Can you work these out from the model? Positions are in its coordinate system, mm. A direction names the side the tool comes from. Round coordinates to 2 decimals unless told otherwise and drop trailing zeros. Order: outer loops, then holes, each group sorted by start corner. A loop starts at its lowest first (then second) coordinate and runs counter-clockwise, first axis right, second up. Notation, with made-up numbers: (24, 53) -> (74, 53) arc R22 cw to (74, 68) -> close; hole circle Ø8 at (43.25, 3). An arc over 180 degrees is marked (long way). One line per item, written item: value.
```python
from build123d import *

# Parameters (mm, degrees)
F1_DEPTH    = 3
F3_DEPTH    = 6
F5_DEPTH    = 12.5
F6_W        = 30
F6_H        = 2.0356480181
F7_DEPTH    = 8
F8_T4_DEPTH = 30
F8_T9_DEPTH = 30


# Not quite as in the source:
# - a fillet or chamfer that OpenCascade refuses, or shapes differently, is made with other operations: its cross-section is extruded or revolved along the edge and cut away or added


with BuildPart() as f1:
    # F0 (on Top) → F1 (new body)
    with BuildSketch(Plane.XY):
        with BuildLine():
            ThreePointArc((22, 30), (20.5355339059, 33.5355339059), (17, 35))
            Line((17, 35), (-17, 35))
            ThreePointArc((-17, 35), (-20.5355339059, 33.5355339059), (-22, 30))
            Line((-22, 30), (-22, -30))
            ThreePointArc((-22, -30), (-20.5355339059, -33.5355339059), (-17, -35))
            Line((-17, -35), (17, -35))
            ThreePointArc((17, -35), (20.5355339059, -33.5355339059), (22, -30))
            Line((22, -30), (22, 30))
        make_face()
    extrude(amount=F1_DEPTH)

    # F2 (on Top) → F3 (join)
    with BuildSketch(Plane.XY):
        with BuildLine():
            ThreePointArc((-12, 30), (-13.4644661049, 33.5355339167), (-17.0000000305, 35))
            ThreePointArc((-17.0000000305, 35), (-20.5355339275, 33.5355338843), (-22, 29.9999999695))
            ThreePointArc((-22, 29.9999999695), (-16.9999999847, 25), (-12, 30))
        make_face()
        with BuildLine():
            ThreePointArc((22, 30), (20.5355339059, 33.5355339059), (17, 35))
            ThreePointArc((17, 35), (13.4644660941, 26.4644660941), (22, 30))
        make_face()
        with BuildLine():
            ThreePointArc((17, -35), (20.5355339059, -33.5355339059), (22, -30))
            ThreePointArc((22, -30), (13.4644660941, -26.4644660941), (17, -35))
        make_face()
        with BuildLine():
            ThreePointArc((-12, -30), (-17, -25), (-22, -30))
            ThreePointArc((-22, -30), (-20.5355339059, -33.5355339059), (-17, -35))
            ThreePointArc((-17, -35), (-13.4644660941, -33.5355339059), (-12, -30))
        make_face()
    extrude(amount=F3_DEPTH)

    # F4 (on Top) → F5 (cut, symmetric)
    with BuildSketch(Plane.XY):
        with BuildLine():
            ThreePointArc((-18.0685374254, -32.3153245497), (-15.6256402281, -32.1479374333), (-14.45, -30))
            ThreePointArc((-14.45, -30), (-14.5093597608, -29.4529979899), (-14.6846754503, -28.9314625746))
            Line((-14.6846754503, -28.9314625746), (-18.0685374254, -32.3153245497))
        make_face()
        with BuildLine():
            Line((-18.0685374254, -32.3153245497), (-14.6846754503, -28.9314625746))
            ThreePointArc((-14.6846754503, -28.9314625746), (-15.196877708, -28.196877708), (-15.9314625746, -27.6846754503))
            Line((-15.9314625746, -27.6846754503), (-19.3153245497, -31.0685374254))
            ThreePointArc((-19.3153245497, -31.0685374254), (-18.803122292, -31.803122292), (-18.0685374254, -32.3153245497))
        make_face()
        with BuildLine():
            ThreePointArc((-15.9314625746, -27.6846754503), (-15.196877708, -28.196877708), (-14.6846754503, -28.9314625746))
            Line((-14.6846754503, -28.9314625746), (-14.16467731, -28.4114644343))
            ThreePointArc((-14.16467731, -28.4114644343), (-14.7019029611, -27.7019029611), (-15.4114644343, -27.16467731))
            Line((-15.4114644343, -27.16467731), (-15.9314625746, -27.6846754503))
        make_face()
        with BuildLine():
            Line((-18.5885355657, -32.83532269), (-18.0685374254, -32.3153245497))
            ThreePointArc((-18.0685374254, -32.3153245497), (-18.803122292, -31.803122292), (-19.3153245497, -31.0685374254))
            Line((-19.3153245497, -31.0685374254), (-19.83532269, -31.5885355657))
            ThreePointArc((-19.83532269, -31.5885355657), (-19.2980970389, -32.2980970389), (-18.5885355657, -32.83532269))
        make_face()
        with BuildLine():
            Line((-19.3153245497, -31.0685374254), (-15.9314625746, -27.6846754503))
            ThreePointArc((-15.9314625746, -27.6846754503), (-18.803122292, -28.196877708), (-19.3153245497, -31.0685374254))
        make_face()
        with BuildLine():
            ThreePointArc((19.3153245497, -31.0685374254), (19.4906402392, -30.5470020101), (19.55, -30))
            ThreePointArc((19.55, -30), (18.3743597719, -27.8520625667), (15.9314625746, -27.6846754503))
            Line((15.9314625746, -27.6846754503), (19.3153245497, -31.0685374254))
        make_face()
        with BuildLine():
            Line((19.3153245497, -31.0685374254), (15.9314625746, -27.6846754503))
            ThreePointArc((15.9314625746, -27.6846754503), (15.196877708, -28.196877708), (14.6846754503, -28.9314625746))
            Line((14.6846754503, -28.9314625746), (18.0685374254, -32.3153245497))
            ThreePointArc((18.0685374254, -32.3153245497), (18.803122292, -31.803122292), (19.3153245497, -31.0685374254))
        make_face()
        with BuildLine():
            ThreePointArc((14.6846754503, -28.9314625746), (15.196877708, -28.196877708), (15.9314625746, -27.6846754503))
            Line((15.9314625746, -27.6846754503), (15.4114644343, -27.16467731))
            ThreePointArc((15.4114644343, -27.16467731), (14.7019029611, -27.7019029611), (14.16467731, -28.4114644343))
            Line((14.16467731, -28.4114644343), (14.6846754503, -28.9314625746))
        make_face()
        with BuildLine():
            Line((19.83532269, -31.5885355657), (19.3153245497, -31.0685374254))
            ThreePointArc((19.3153245497, -31.0685374254), (18.803122292, -31.803122292), (18.0685374254, -32.3153245497))
            Line((18.0685374254, -32.3153245497), (18.5885355657, -32.83532269))
            ThreePointArc((18.5885355657, -32.83532269), (19.2980970389, -32.2980970389), (19.83532269, -31.5885355657))
        make_face()
        with BuildLine():
            Line((18.0685374254, -32.3153245497), (14.6846754503, -28.9314625746))
            ThreePointArc((14.6846754503, -28.9314625746), (15.196877708, -31.803122292), (18.0685374254, -32.3153245497))
        make_face()
        with BuildLine():
            ThreePointArc((15.9314625746, 27.6846754503), (18.3743597719, 27.8520625667), (19.55, 30))
            ThreePointArc((19.55, 30), (19.4906402392, 30.5470020101), (19.3153245497, 31.0685374254))
            Line((19.3153245497, 31.0685374254), (15.9314625746, 27.6846754503))
        make_face()
        with BuildLine():
            Line((15.9314625746, 27.6846754503), (19.3153245497, 31.0685374254))
            ThreePointArc((19.3153245497, 31.0685374254), (18.803122292, 31.803122292), (18.0685374254, 32.3153245497))
            Line((18.0685374254, 32.3153245497), (14.6846754503, 28.9314625746))
            ThreePointArc((14.6846754503, 28.9314625746), (15.196877708, 28.196877708), (15.9314625746, 27.6846754503))
        make_face()
        with BuildLine():
            ThreePointArc((18.0685374254, 32.3153245497), (18.803122292, 31.803122292), (19.3153245497, 31.0685374254))
            Line((19.3153245497, 31.0685374254), (19.83532269, 31.5885355657))
            ThreePointArc((19.83532269, 31.5885355657), (19.2980970389, 32.2980970389), (18.5885355657, 32.83532269))
            Line((18.5885355657, 32.83532269), (18.0685374254, 32.3153245497))
        make_face()
        with BuildLine():
            Line((15.4114644343, 27.16467731), (15.9314625746, 27.6846754503))
            ThreePointArc((15.9314625746, 27.6846754503), (15.196877708, 28.196877708), (14.6846754503, 28.9314625746))
            Line((14.6846754503, 28.9314625746), (14.16467731, 28.4114644343))
            ThreePointArc((14.16467731, 28.4114644343), (14.7019029611, 27.7019029611), (15.4114644343, 27.16467731))
        make_face()
        with BuildLine():
            Line((14.6846754503, 28.9314625746), (18.0685374254, 32.3153245497))
            ThreePointArc((18.0685374254, 32.3153245497), (15.196877708, 31.803122292), (14.6846754503, 28.9314625746))
        make_face()
        with BuildLine():
            ThreePointArc((-14.6846754503, 28.9314625746), (-14.5093597608, 29.4529979899), (-14.45, 30))
            ThreePointArc((-14.45, 30), (-15.6256402281, 32.1479374333), (-18.0685374254, 32.3153245497))
            Line((-18.0685374254, 32.3153245497), (-14.6846754503, 28.9314625746))
        make_face()
        with BuildLine():
            Line((-14.6846754503, 28.9314625746), (-18.0685374254, 32.3153245497))
            ThreePointArc((-18.0685374254, 32.3153245497), (-18.803122292, 31.803122292), (-19.3153245497, 31.0685374254))
            Line((-19.3153245497, 31.0685374254), (-15.9314625746, 27.6846754503))
            ThreePointArc((-15.9314625746, 27.6846754503), (-15.196877708, 28.196877708), (-14.6846754503, 28.9314625746))
        make_face()
        with BuildLine():
            ThreePointArc((-19.3153245497, 31.0685374254), (-18.803122292, 31.803122292), (-18.0685374254, 32.3153245497))
            Line((-18.0685374254, 32.3153245497), (-18.5885355657, 32.83532269))
            ThreePointArc((-18.5885355657, 32.83532269), (-19.2980970389, 32.2980970389), (-19.83532269, 31.5885355657))
            Line((-19.83532269, 31.5885355657), (-19.3153245497, 31.0685374254))
        make_face()
        with BuildLine():
            Line((-14.16467731, 28.4114644343), (-14.6846754503, 28.9314625746))
            ThreePointArc((-14.6846754503, 28.9314625746), (-15.196877708, 28.196877708), (-15.9314625746, 27.6846754503))
            Line((-15.9314625746, 27.6846754503), (-15.4114644343, 27.16467731))
            ThreePointArc((-15.4114644343, 27.16467731), (-14.7019029611, 27.7019029611), (-14.16467731, 28.4114644343))
        make_face()
        with BuildLine():
            Line((-15.9314625746, 27.6846754503), (-19.3153245497, 31.0685374254))
            ThreePointArc((-19.3153245497, 31.0685374254), (-18.803122292, 28.196877708), (-15.9314625746, 27.6846754503))
        make_face()
    extrude(amount=F5_DEPTH, both=True, mode=Mode.SUBTRACT)

    # F6 (on Top) → F7 (join)
    with BuildSketch(Plane.XY):
        with Locations((0, 23.2678240091)):
            Rectangle(F6_W, F6_H)
        with Locations((0, -23.2678240091)):
            Rectangle(F6_W, F6_H)
    extrude(amount=F7_DEPTH)

    # F8: chamfer of 5 x 2 on 2 edges, made by hand


with BuildPart() as f8_tool2:
    # F8_s3 → F8_t4 (new body)
    with BuildSketch(Plane.YZ.offset(-15)):
        Polygon((26.2856480181, 3), (24.2856480181, 8), (24.2856480181, 3), align=None)
    extrude(amount=F8_T4_DEPTH)

    split(bisect_by=Plane.XY.offset(8), keep=Keep.BOTTOM)


with BuildPart() as f1_1:
    add(f1.part)

    # F8_t1: union F8_tool2
    add(f8_tool2.part)


with BuildPart() as f8_tool7:
    # F8_s8 → F8_t9 (new body)
    with BuildSketch(Plane.YZ.offset(15)):
        Polygon((-26.2856480181, 3), (-24.2856480181, 8), (-24.2856480181, 3), align=None)
    extrude(amount=-F8_T9_DEPTH)

    split(bisect_by=Plane.XY.offset(8), keep=Keep.BOTTOM)


with BuildPart() as f1_2:
    add(f1_1.part)

    # F8_t6: union F8_tool7
    add(f8_tool7.part)


solid = f1_2.part
```
Q1. I want a section at A-A on x = 7. List the corners of the cut face in (y, z) for me.
Answers below:
outline: (-35, 0) -> (35, 0) -> (35, 3) -> (26.29, 3) -> (24.29, 8) -> (22.25, 8) -> (22.25, 3) -> (-22.25, 3) -> (-22.25, 8) -> (-24.29, 8) -> (-26.29, 3) -> (-35, 3) -> close
Q2. On a 3-axis mill with a long thin cutter (end or side, diameter ignored), from which of +Z, -Z, +X, -X, +Y, -Y can I reach the whole of each face in a straight line? I mean faces 1 (the face through (-14.711, 27.693, 3.042)), 2 (the face through (0, -23, 8)). Say none if no direction works.
Answers below:
face 1: +Z, -Z
face 2: +Z, +X, -X, +Y, -Y
Q3. Please list where these lines run through material, in increasing order: line 1 along Y through (x, z) = (-17, 3.5); line 2 along X through (y, z) = (31, 4.5); line 3 along Z through (x, y) = (5, 3).
Answers below:
line 1: -35 to -32.55, -27.45 to -25, 25 to 27.45, 32.55 to 35
line 2: -21.9 to -19.35, -14.65 to -12.1, 12.1 to 14.65, 19.35 to 21.9
line 3: 0 to 3
Q4. Will these pins go through, and if not, where does the flat tip stop? pin 1 Ø2.5 at (y, z) = (24.5, 4.5) entering from +X; pin 2 Ø1.5 at (x, z) = (5, 4) entering from -Y; pin 3 Ø4 at (x, y) = (3.5, 11) entering from +Z.
Answers below:
pin 1: x = 19.63
pin 2: y = -26.19
pin 3: z = 3
Q5. We'd pull the mould along X, two halves only. Please class faces 3 (the face through (-22, 0, 1)), 4 (the face through (0, 0, 0)), 5 (the face through (-21, 33, 4)): released by +X, released by -X, zero draft, split by the parting line, or undercut.
Answers below:
face 3: released by -X
face 4: zero draft
face 5: undercut
Q6. I want a section at C-C on y = -15. List the corners of the cut face in (x, z) for me.
Answers below:
outline: (-22, 0) -> (22, 0) -> (22, 3) -> (-22, 3) -> close
Q7. I want a section at B-B on z = 7. List the corners of the cut face in (x, y) for me.
Answers below:
outline: (-15, -24.69) -> (15, -24.69) -> (15, -22.25) -> (-15, -22.25) -> close; (-15, 22.25) -> (15, 22.25) -> (15, 24.69) -> (-15, 24.69) -> close
